from build123d import *

# Parameters (mm, degrees)
F0_R     = 11.5
F1_DEPTH = 13.5
F2_SIZE  = 1


with BuildPart() as f1:
    # F0 (on Top) → F1 (new body)
    with BuildSketch(Plane.XY):
        Polygon((14, -3.751289), (14, 3.751289), (10.248711, 10.248711), (3.751289, 14), (-3.751289, 14), (-10.248711, 10.248711), (-14, 3.751289), (-14, -3.751289), (-10.248711, -10.248711), (-3.751289, -14), (3.751289, -14), (10.248711, -10.248711), align=None)
        Circle(F0_R, mode=Mode.SUBTRACT)
    extrude(amount=F1_DEPTH)

    # F2
    f2_edges = [f1.edges().sort_by_distance(p)[0] for p in [
        (7, -12.124356, 13.5),
        (14, 0, 13.5),
        (12.124356, 7, 13.5),
        (7, 12.124356, 13.5),
        (0, 14, 13.5),
        (-7, 12.124356, 13.5),
        (-12.124356, 7, 13.5),
        (-14, 0, 13.5),
        (-12.124356, -7, 13.5),
        (-7, -12.124356, 13.5),
        (0, -14, 13.5),
        (14, 0, 0),
        (12.124356, 7, 0),
        (7, 12.124356, 0),
        (0, 14, 0),
        (-7, 12.124356, 0),
        (-12.124356, 7, 0),
        (-14, 0, 0),
        (-12.124356, -7, 0),
        (-7, -12.124356, 0),
        (0, -14, 0),
        (7, -12.124356, 0),
        (12.124356, -7, 0),
        (12.124356, -7, 13.5),
    ]]
    chamfer(f2_edges, length=F2_SIZE)


solid = f1.part
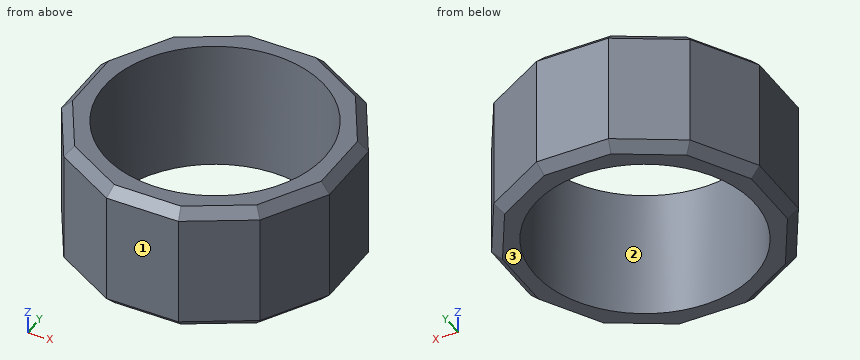
Read the model definition and answer for the solid it produces. Units are mm, in the model's axes. Face numbers are marked on the shaded views. Round coordinates to 2 decimals unless told otherwise and drop trailing zeros. Order: outer loops, then holes, each group sorted by start corner. A loop starts at its lowest first (then second) coordinate and runs counter-clockwise, first axis right, second up.
1) The part is cut by section B-B on z = 2.5. Write down the section's boundary in (x, y), plus the area to 3 significant figures.
2) Straight lines are drawn through the part: L1, parallel to Y at x = 0, z = 3.5; L2, parallel to X at y = 4.5, z = 4. For each, find the intervals that lie inside material, in ascending order.
3) Flat-ended cylindrical pins translate along their axes: pin 1 (1 mm diameter, centred on x = -8.5, z = 4.5, fed in from +Y); pin 2 (1 mm diameter, centred on y = -11, z = 4.5, fed in from +X); pin 3 (2 mm diameter, centred on x = -9, z = 5.5, fed in from -Y). Find the tip coordinate at first contact, or state that the pin passes through.
4) The mould has two halves that part along Y. Classify the marked faces 1, 2 and 3: released by +Y, released by -Y, zero draft, split by the parting line, or undercut.
5) The part is cut by section A-A on x = 0. Write down the section's boundary in (y, z), plus the area to 3 significant figures.
Resolved:
1. outline: (-14, -3.75) - (-10.25, -10.25) - (-3.75, -14) - (3.75, -14) - (10.25, -10.25) - (14, -3.75) - (14, 3.75) - (10.25, 10.25) - (3.75, 14) - (-3.75, 14) - (-10.25, 10.25) - (-14, 3.75) - close; hole circle Ø23 at (0, 0)
1. area: 215 mm2
2. L1: y = -14 to -11.5, 11.5 to 14
2. L2: x = -13.57 to -10.58, 10.58 to 13.57
3. pin 1: stops at y = 11.55
3. pin 2: stops at x = 9.81
3. pin 3: stops at y = -11.55
4. face 1: released by -Y
4. face 2: undercut
4. face 3: zero draft
5. outline: (-14, 1) - (-13, 0) - (-11.5, 0) - (-11.5, 13.5) - (-13, 13.5) - (-14, 12.5) - close; (11.5, 0) - (13, 0) - (14, 1) - (14, 12.5) - (13, 13.5) - (11.5, 13.5) - close
5. area: 65.5 mm2
